Verification items for the finished model (mm, model axes). A direction names the side the tool comes from. Coordinates: 2 decimals unless noted, no trailing zeros. Order: outer loops, then holes, each group sorted by start corner. A loop starts at its lowest first (then second) coordinate and runs counter-clockwise, first axis right, second up. Notation, with made-up numbers: M 27,15 L 33,15 A13 cw 33,20 Z; hole C 1,81 d11. An arc over 180 degrees is marked long. Return JSON: item names as keys, results as strings. Group by question number.
1. Section check A-A, the plane x = 0. Record the cut outline in (y, z).
2. Section check D-D, the plane z = 30.5. Record the cut outline in (x, y), plus the area to 3 significant figures.
3. Material ranges on line 1 along X through (y, z) = (-0.05, 16); line 2 along Y through (x, z) = (-0.9, 1); line 3 along Z through (x, y) = (-1.15, -0.15), recorded low to high.
4. Section check C-C, the plane z = 9.5. Record the cut outline in (x, y).
5. Set-up check for faces 1 (the flat face through (0, 0, 32)), 2 (the cylindrical face through (0, -1, 22)): record each of +Z, -Z, +X, -X, +Y, -Y from which the full face is reachable in a straight line by a thin tool's end or side.
```python
from build123d import *

# Parameters (mm, degrees)
SKETCH1_R           = 1.5
BOSS_EXTRUDE1_DEPTH = 12
SKETCH2_R           = 1
BOSS_EXTRUDE2_DEPTH = 20
CHAMFER1_SIZE       = 0.3
CHAMFER2_SIZE       = 0.1


with BuildPart() as part:
    # Sketch1 → Boss-Extrude1 (new body)
    with BuildSketch(Plane.XY):
        Circle(SKETCH1_R)
    extrude(amount=BOSS_EXTRUDE1_DEPTH)

    # Sketch2 → Boss-Extrude2 (add)
    with BuildSketch(Plane.XY.offset(12)):
        Circle(SKETCH2_R)
    extrude(amount=BOSS_EXTRUDE2_DEPTH)

    # Chamfer1
    chamfer1_edges = [part.edges().sort_by_distance(p)[0] for p in [
        (-1.5, 0, 0),
    ]]
    chamfer(chamfer1_edges, length=CHAMFER1_SIZE)

    # Chamfer2
    chamfer2_edges = [part.edges().sort_by_distance(p)[0] for p in [
        (-1, 0, 12),
        (-1, 0, 32),
    ]]
    chamfer(chamfer2_edges, length=CHAMFER2_SIZE)


solid = part.part
```
Answers follow:
{
 "1": {"outline": "M -1.5,0.3 L -1.2,0 L 1.2,0 L 1.5,0.3 L 1.5,12 L 1.1,12 L 1,12.1 L 1,31.9 L 0.9,32 L -0.9,32 L -1,31.9 L -1,12.1 L -1.1,12 L -1.5,12 Z"},
 "2": {"outline": "C 0,0 d2", "area": "3.14 mm^2"},
 "3": {"line 1": "-1 to 1", "line 2": "-1.2 to 1.2", "line 3": "0 to 12"},
 "4": {"outline": "C 0,0 d3"},
 "5": {"face 1": "+Z, +X, -X, +Y, -Y", "face 2": "+Z"}
}
